Autodesk Inventor part; units mm, degrees
ref_plane "YZ Plane" through (0, 0, 0) normal (1, 0, 0) x (0, 1, 0)
ref_plane "XZ Plane" through (0, 0, 0) normal (0, 1, 0) x (-1, 0, 0)
ref_plane "XY Plane" through (0, 0, 0) normal (0, 0, 1) x (1, 0, 0)
sketch "Skizze1" plane through (0, 0, 0) normal (0, 1, 0) x (-1, 0, 0)
  line L0 (0, 0) -> (-48, 0)
  line L1 (-48, 0) -> (-48, -102)
  line L2 (-48, -102) -> (-34, -102)
  line L3 (-34, -102) -> (-34, -52)
  line L4 (-34, -52) -> (-46, -52)
  line L5 (-46, -52) -> (-46, -2)
  line L6 (-46, -2) -> (0, -2)
  line L7 (0, -2) -> (0, 0)
  dimension "d0" = 2
  dimension "d1" = 46
  dimension "d2" = 48
  dimension "d3" = 50
  dimension "d4" = 50
  dimension "d5" = 12
extrude "Extrusion1" add sketch "Skizze1" along normal blind 25
sketch "Skizze2" plane through (0, 25, 0) normal (0, 1, 0) x (1, 0, 0)
  line L0 (48, 0) -> (48, 102)
  line L1 (48, 102) -> (34, 102)
  line L2 (34, 102) -> (34, 52)
  line L3 (34, 52) -> (46, 52)
  line L4 (46, 52) -> (46, 2)
  line L5 (46, 2) -> (0, 2)
  line L6 (0, 2) -> (0, 0)
  line L7 (0, 0) -> (48, 0)
  line L8 (46, 59) -> (46, 95)
  line L9 (46, 95) -> (41, 95)
  line L10 (41, 95) -> (41, 90)
  line L11 (41, 90) -> (34, 90)
  line L12 (34, 64) -> (38, 64)
  line L13 (38, 64) -> (38, 59)
  line L14 (38, 59) -> (46, 59)
  point P0 (34, 77)
  point P1 (46, 77)
  point P2 (39, 59)
  dimension "d18" = 5
  dimension "d19" = 36
  dimension "d20" = 5
  dimension "d21" = 8
  dimension "d22" = 5
extrude "Extrusion2" cut sketch "Skizze2" against normal through all contours L11 L10 L9 L8 L14 L13 L12 L2
sketch "Skizze3" plane through (34, 0, -52) normal (0, 0, 1) x (1, 0, 0)
  line L0 (0, 0) -> (12, 0)
  line L1 (12, 0) -> (12, 25)
  line L2 (0, 25) -> (12, 25)
  line L3 (0, 0) -> (0, 25)
  line L4 (12, 0) -> (12, 25)
  line L5 (12, 6.25) -> (0, 6.25)
  line L6 (0, 0) -> (0, 25)
  line L7 (0, 18.75) -> (12, 18.75)
  line L8 (6, 6.25) -> (6, 18.75) construction
  point P0 (-34, 0)
  point P1 (6, 12.5)
  point P2 (0, 12.5)
  dimension "d15" = 12.5
extrude "Extrusion3" cut sketch "Skizze3" against normal up to surface (12 mm away) contours L3 L7 L1 L5
properties part number "ESP_stand"
For this review, take the finished solid that the model builds, in its own axes (mm). A direction names the side the tool comes from. Round coordinates to 2 decimals unless told otherwise and drop trailing zeros. Order: outer loops, then holes, each group sorted by start corner. A loop starts at its lowest first (then second) coordinate and runs counter-clockwise, first axis right, second up.
Q1. We need section D-D, the plane x = 4. Give the boundary of the cut face in (y, z), plus the area to 3 significant figures.
Findings below:
outline: (0, -2) - (25, -2) - (25, 0) - (0, 0) - close
area: 50.0 mm2
Q2. We need section B-B, the plane z = -61. Give the boundary of the cut face in (x, y).
Findings below:
outline: (34, 0) - (38, 0) - (38, 6.25) - (34, 6.25) - close; (34, 18.75) - (38, 18.75) - (38, 25) - (34, 25) - close; (46, 0) - (48, 0) - (48, 25) - (46, 25) - close
Q3. Wall thickness on line 1 (Z direction, x = 37.5, y = 23); line 2 (Z direction, x = 39.5, y = 15); line 3 (Y direction, x = 43.5, z = -55): over which ranges is each line inside the solid? List them lowest first.
Findings below:
line 1: z = -102 to -90, -64 to -52, -2 to 0
line 2: z = -102 to -90, -2 to 0
line 3: y = 0 to 6.25, 18.75 to 25
Q4. Insertion check: P1, Ø3.5, axis at y = 14, z = -98.5, coming from the -X side; P2, Ø7.5, axis at y = 17, z = -30, coming from the -X side; P3, Ø7.5, axis at x = 13, y = 16.5, coming from the -Z side. Each pin has a flat end and moves straight along its axis. Give the tip position at first contact, or say it passes through.
Findings below:
P1: stops at x = 34
P2: stops at x = 46
P3: stops at z = -2
Q5. We need section C-C, the plane y = 8. Give the boundary of the cut face in (x, z).
Findings below:
outline: (0, -2) - (46, -2) - (46, -95) - (41, -95) - (41, -90) - (34, -90) - (34, -102) - (48, -102) - (48, 0) - (0, 0) - close
Q6. We need section A-A, the plane x = 39.5. Give the boundary of the cut face in (y, z).
Findings below:
outline: (0, -102) - (25, -102) - (25, -90) - (0, -90) - close; (0, -59) - (6.25, -59) - (6.25, -52) - (0, -52) - close; (0, -2) - (25, -2) - (25, 0) - (0, 0) - close; (18.75, -59) - (25, -59) - (25, -52) - (18.75, -52) - close
Q7. Mouldability with a two-part tool opening along X and no side actions: class faces 1 (the flat face through (38, 13, -90)), 2 (the flat face through (41, 13, -93)), 3 (the flat face through (34, 22, -58)), 4 (the flat face through (48, 12, -50)) as pulls with the +X half, pulls with the -X half, needs draft (parallel to the pull), parting line crosses it, or undercut.
Findings below:
face 1: needs draft
face 2: undercut
face 3: pulls with the -X half
face 4: pulls with the +X half
Q8. Machinability: for faces 5 (the flat face through (34, 3, -58)), 6 (the flat face through (38, 3, -62)), 7 (the flat face through (39, 6.25, -57)), 8 (the flat face through (36, 22, -64)), which of the approach directions +Z, -Z, +X, -X, +Y, -Y give a long, thin tool a straight path to every point of the face, cutting with its end or side? Answer none if there is none.
Findings below:
face 5: -Z, -X, +Y, -Y
face 6: +Y, -Y
face 7: -X
face 8: -X, +Y, -Y
